Verification items for the finished model (mm, model axes). A direction names the side the tool comes from. Give positions to 0.01 mm unless a question says otherwise; leave off trailing zeros. Order: outer loops, then holes, each group sorted by start corner. A loop starts at its lowest first (then second) coordinate and runs counter-clockwise, first axis right, second up.
(1) Scan lines: L1, parallel to X at y = -9, z = -22; L2, parallel to Y at x = -17.5, z = -14.5; L3, parallel to Z at x = -12.5, y = 6.5. Record each from-to range of solid material in increasing order.
(2) Sectioned sample at C-C on z = -48.5. Record the cut outline in (x, y).
(3) Sectioned sample at B-B on x = 0. Record the cut outline in (y, z).
(4) Sectioned sample at A-A on y = -11. Record the cut outline in (x, z).
(5) Sectioned sample at D-D on y = -18. Record the cut outline in (x, z).
(6) Access from +Z, -Z, +X, -X, +Y, -Y to the whole of each face (thin tool, end or side, straight path). Record for faces 4 (the face through (-27.899, 3.656, -14.454)), 5 (the face through (-3.677, -10, -13)), 6 (the face through (-12.1, -9.9, -36)), 7 (the face through (-25, 0, -17)).
(7) Mould release check, pull along Z, two halves, no side actions. Record for faces 1 (the face through (-51.421, -5.21, -8.345)), 2 (the face through (57.43, 10.25, -47.54)), 3 (the face through (23.89, 4.25, -71.59)): pulls with the +Z half, pulls with the -Z half, needs draft (parallel to the pull), parting line crosses it, or undercut.
(8) Gauge pin test, flat ends, axial feed: pin 1 (2 mm diameter, centred on y = -8, z = -10.5, fed in from +X); pin 2 (1.5 mm diameter, centred on x = -19, y = 2, fed in from -Z); pin 3 (4 mm diameter, centred on y = -8.5, z = -69, fed in from +X); pin 4 (2.5 mm diameter, centred on x = 46.29, z = -10.25, fed in from -Y). Record the tip position at first contact, or that the pin passes through.
```python
from build123d import *

# Parameters (mm, degrees)
SKETCH1_R                                            = 1.0000000000000018
SKETCH1_R_2                                          = 1.0000000000000087
SKETCH1_R_3                                          = 0.9999999999999911
SKETCH1_R_4                                          = 1.000000000000005
SKETCH1_R_5                                          = 0.9999999999999983
MAIN_BODY_DEPTH                                      = 10.5
PROFILE_STOPS_DEPTH                                  = 20
CSK_FOR_M3_HEX_SOCKET_COUNTERSUNK_HEAD_S_D           = 3.2
CSK_FOR_M3_HEX_SOCKET_COUNTERSUNK_HEAD_S_DEPTH       = 30.5
CSK_FOR_M3_HEX_SOCKET_COUNTERSUNK_HEAD_S_CSINK_D     = 6.94
CSK_FOR_M3_HEX_SOCKET_COUNTERSUNK_HEAD_S_CSINK_ANGLE = 90
CSK_FOR_M5_HEX_SOCKET_COUNTERSUNK_HEAD_S_D           = 5.3
CSK_FOR_M5_HEX_SOCKET_COUNTERSUNK_HEAD_S_DEPTH       = 30.5
CSK_FOR_M5_HEX_SOCKET_COUNTERSUNK_HEAD_S_CSINK_D     = 11.47
CSK_FOR_M5_HEX_SOCKET_COUNTERSUNK_HEAD_S_CSINK_ANGLE = 90
FILLET1_R                                            = 5
FILLET3_R                                            = 5
FILLET4_R                                            = 13
DRAFT1_ANGLE                                         = 0.5000000000000011
CHAMFER1_SIZE                                        = 0.5


with BuildPart() as part:
    # Sketch1 → Main Body (new body)
    with BuildSketch(Plane(origin=(0, 0, 0), x_dir=(1, 0, 0), z_dir=(0, 1, 0))):
        Polygon((-75, 0), (75, 2.755e-14), (39.90666646784656, 96.41814145298106), align=None)
        with Locations(Location((-28.015368960704585, 17.101007166283473, 0), (0, 0, 90))):
            Circle(SKETCH1_R, mode=Mode.SUBTRACT)
        with Locations(Location((21.305293098803567, 10.25, 0), (0, 0, 90))):
            Circle(SKETCH1_R_2, mode=Mode.SUBTRACT)
        with Locations(Location((46.28729909878749, 10.25, 0), (0, 0, 90))):
            Circle(SKETCH1_R_3, mode=Mode.SUBTRACT)
        with Locations(Location((5.362707620569896, 54.05189360917208, 0), (0, 0, 90))):
            Circle(SKETCH1_R_4, mode=Mode.SUBTRACT)
        with Locations(Location((24.500034494822536, 70.11001753107655, 0), (0, 0, 90))):
            Circle(SKETCH1_R_5, mode=Mode.SUBTRACT)
    extrude(amount=MAIN_BODY_DEPTH)

    # Sketch1<3> → Profile Stops (add)
    with BuildSketch(Plane(origin=(0, 0, 0), x_dir=(1, 0, 0), z_dir=(0, 1, 0))):
        Polygon((-75, 0), (-3.676712901180352, 1.84e-15), (-3.67671290118036, 20.5), (67.53861019754284, 20.5), (47.36805627030374, 75.91814145298105), (-7.186046254395704, 30.141814145298103), (-20.363192252969785, 45.84572522923713), align=None)
        Polygon((-41.15292479284825, 23.22715006025093), (-21.889226066737145, 30.238562998427152), (-14.877813128560916, 10.974864272316022), (-34.14151185467204, 3.9634513341398048), align=None, mode=Mode.SUBTRACT)
    extrude(amount=-PROFILE_STOPS_DEPTH)

    # CSK for M3 Hex Socket Countersunk Head Screw1
    with Locations(Plane(origin=(24.500034495, 10.5, -70.110017531), x_dir=(0, 0, 1), z_dir=(0, 1, 0))):
        with Locations((0, 0), (16.058123922, -19.137326874), (59.860017531, 21.787264604), (59.860017531, -3.194741396)):
            CounterSinkHole(CSK_FOR_M3_HEX_SOCKET_COUNTERSUNK_HEAD_S_D / 2, CSK_FOR_M3_HEX_SOCKET_COUNTERSUNK_HEAD_S_CSINK_D / 2, depth=CSK_FOR_M3_HEX_SOCKET_COUNTERSUNK_HEAD_S_DEPTH, counter_sink_angle=CSK_FOR_M3_HEX_SOCKET_COUNTERSUNK_HEAD_S_CSINK_ANGLE)

    # CSK for M5 Hex Socket Countersunk Head Screw1
    with Locations(Plane(origin=(-28.015368961, 10.5, -17.101007166), x_dir=(0, 0, 1), z_dir=(0, 1, 0))):
        with Locations((0, 0)):
            CounterSinkHole(CSK_FOR_M5_HEX_SOCKET_COUNTERSUNK_HEAD_S_D / 2, CSK_FOR_M5_HEX_SOCKET_COUNTERSUNK_HEAD_S_CSINK_D / 2, depth=CSK_FOR_M5_HEX_SOCKET_COUNTERSUNK_HEAD_S_DEPTH, counter_sink_angle=CSK_FOR_M5_HEX_SOCKET_COUNTERSUNK_HEAD_S_CSINK_ANGLE)

    # Fillet1
    fillet1_edges = [part.edges().sort_by_distance(p)[0] for p in [
        (-3.676712901180355, -10, -2.69e-15),
        (-20.363192252969785, -10, -45.84572522923713),
    ]]
    fillet(fillet1_edges, radius=FILLET1_R)

    # Fillet3
    fillet3_edges = [part.edges().sort_by_distance(p)[0] for p in [
        (75, 5.25, -2.755e-14),
        (39.90666646784656, 5.25, -96.41814145298106),
        (47.36805627030374, -10, -75.91814145298105),
        (67.53861019754285, -10, -20.5),
    ]]
    fillet(fillet3_edges, radius=FILLET3_R)

    # Fillet4
    fillet4_edges = [part.edges().sort_by_distance(p)[0] for p in [
        (-75, -4.75, 0),
    ]]
    fillet(fillet4_edges, radius=FILLET4_R)

    # Draft1
    draft1_faces = [part.faces().sort_by_distance(p)[0] for p in [
        (-31.521075429792702, -10, -26.732856529339042),
        (-18.38351959764903, -10, -20.606713635371584),
        (-37.64721832376015, -10, -13.59530069719537),
        (-24.509662491616478, -10, -7.469157803227914),
    ]]
    draft(draft1_faces, Plane(origin=(0, 0, 0), x_dir=(0, 0, -1), z_dir=(0, -1, 0)), DRAFT1_ANGLE)

    # Chamfer1
    chamfer1_edges = [part.edges().sort_by_distance(p)[0] for p in [
        (57.45333323392328, 10.5, -48.209070726490545),
        (38.94457551921066, 10.5, -92.82756915116973),
        (71.9550201877344, 10.5, -2.1321178182447977),
        (14.288233209599724, 10.5, -1.64e-14),
        (-6.601245113874818, 10.5, -57.39336999793299),
        (-51.498797617306785, 10.5, -8.553738136766313),
    ]]
    chamfer(chamfer1_edges, length=CHAMFER1_SIZE)


solid = part.part
```
Ans:
1. L1: x = -48.66 to -40.79, -18.81 to 63.97
1. L2: y = 0 to 10.5
1. L3: z = -52.44 to 0
2. outline: (-17.2, 0) - (14.69, 0) - (14.69, -20) - (57.35, -20) - (57.35, 10) - (56.82, 10.5) - (-16.42, 10.5) - (-17.2, 10) - close
3. outline: (-20, -36.17) - (0, -36.17) - (0, -62.93) - (10, -62.93) - (10.5, -62.28) - (10.5, -0.5) - (10, 0) - (0, 0) - (0, -20.5) - (-20, -20.5) - close
4. outline: (-47.64, -22.96) - (-24.19, -42.63) arc R5 ccw to (-17.15, -42.02) - (-7.19, -30.14) - (41.9, -71.33) arc R5 ccw to (49.81, -69.21) - (65.1, -27.21) arc R5 ccw to (60.4, -20.5) - (-3.68, -20.5) - (-3.68, -5) arc R5 ccw to (-8.68, 0) - (-39.28, 0) arc R13 ccw to start; hole (-41.28, -23.28) - (-21.83, -30.36) - (-14.75, -10.92) - (-34.2, -3.84) - close
5. outline: (-47.64, -22.96) - (-24.19, -42.63) arc R5 ccw to (-17.15, -42.02) - (-7.19, -30.14) - (41.9, -71.33) arc R5 ccw to (49.81, -69.21) - (65.1, -27.21) arc R5 ccw to (60.4, -20.5) - (-3.68, -20.5) - (-3.68, -5) arc R5 ccw to (-8.68, 0) - (-39.28, 0) arc R13 ccw to start; hole (-41.35, -23.32) - (-21.8, -30.44) - (-14.68, -10.88) - (-34.24, -3.76) - close
6. face 4: +Y, -Y
6. face 5: +Z, +X, -Y
6. face 6: -Z, -Y
6. face 7: -Y
7. face 1: parting line crosses it
7. face 2: pulls with the -Z half
7. face 3: undercut
8. pin 1: stops at x = -3.68
8. pin 2: stops at z = -47.62
8. pin 3: stops at x = 50.61
8. pin 4: passes through
